```python
from build123d import *

# Parameters (mm, degrees)
F1_DEPTH = 28
F3_DEPTH = 72
F5_DEPTH = 28
F6_R     = 2
F7_R     = 1
F8_R     = 4.25
F9_DEPTH = 25


with BuildPart() as f1:
    # F0 (on Top) → F1 (new body)
    with BuildSketch(Plane.XY):
        Polygon((-19.75, -17.750001), (-19.75, -19.75), (-9.25, -19.75), (19.75, 9.25), (19.75, 19.75), (17.750001, 19.75), (17.750001, 10.078427), (-10.078427, -17.750001), align=None)
    extrude(amount=F1_DEPTH)

    # F2 (on face) → F3 (join)
    with BuildSketch(Plane.XY.offset(28)):
        Polygon((-19.75, -19.75), (-9.25, -19.75), (19.75, 9.25), (19.75, 19.75), (11.25, 19.75), (11.25, 24.25), (9.25, 26.25), (9.25, 23.421573), (9.25, 19.75), (9.25, 17.750001), (17.750001, 17.750001), (17.750001, 10.078427), (16.585787, 8.914213), (-8.914213, -16.585787), (-10.078427, -17.750001), (-17.750001, -17.750001), (-17.750001, -9.25), (-19.75, -9.25), (-23.421573, -9.25), (-26.25, -9.25), (-24.25, -11.25), (-19.75, -11.25), align=None)
    extrude(amount=F3_DEPTH)

    # F4 (on face) → F5 (join)
    with BuildSketch(Plane.XY.offset(100)):
        Polygon((19.75, 9.25), (19.75, 19.75), (17.750001, 19.75), (17.750001, 10.078427), (-10.078427, -17.750001), (-19.75, -17.750001), (-19.75, -19.75), (-9.25, -19.75), align=None)
    extrude(amount=F5_DEPTH)

    # F6
    f6_edges = [f1.edges().sort_by_distance(p)[0] for p in [
        (19.75, 9.25, 64),
        (-9.25, -19.75, 64),
    ]]
    fillet(f6_edges, radius=F6_R)

    # F7
    f7_edges = [f1.edges().sort_by_distance(p)[0] for p in [
        (-19.75, -19.75, 64),
        (19.75, 19.75, 64),
    ]]
    fillet(f7_edges, radius=F7_R)

    # F8 (on face) → F9 (cut)
    with BuildSketch(Plane(origin=(5.25, -5.25, 0), x_dir=(0.707107, 0.707107, 0), z_dir=(0.707107, -0.707107, 0))):
        with Locations((0, 114)):
            Circle(F8_R)
    extrude(amount=-F9_DEPTH, mode=Mode.SUBTRACT)


solid = f1.part
```
Check sheet for the modelled part. Datum: model origin and axes. Units: mm. A direction names the side the tool comes from. Round coordinates to 2 decimals unless told otherwise and drop trailing zeros. Write each loop counter-clockwise with the first axis right and the second up, starting at its lowest first coordinate (ties: lowest second). Pieces come first, ordered by that corner, then holes. Notation, with made-up numbers: (-33.5, 72.5) -> (-6.5, 72.5) arc R15 cw to (-6.5, 78.5) -> close; hole circle Ø3 at (39.5, 48). An arc over 180 degrees is marked (long way). Put each result on its own line as item: value.
(1) Sectioned sample at D-D (x = -16). Enter the section's corners in (y, z).
Values found:
outline: (-19.75, 0) -> (-17.75, 0) -> (-17.75, 128) -> (-19.75, 128) -> close
(2) Go/stop test with flat-tipped pins: pin 1 Ø9.5 at (y, z) = (-14, 53.5) entering from +X; pin 2 Ø5 at (x, z) = (-3, 88.5) entering from +Y; pin 3 Ø10.5 at (y, z) = (14.5, 69.5) entering from -X; pin 4 Ø8 at (x, y) = (11.5, 12) entering from -Z. Record where each tip stops, or that it passes through.
Values found:
pin 1: stops at x = 1.25
pin 2: stops at y = -8.17
pin 3: stops at x = 9.25
pin 4: passes through
(3) Tool access check on faces 5 (the face through (-19.75, -15, 63)), 6 (the face through (12.2, 19.5, 100)), 7 (the face through (11.25, 22, 63)). Record the directions out of +Z, -Z, +X, -X, +Y, -Y that give a thin tool (end or side, any length) a straight path to the whole face; none if there is none.
Values found:
face 5: +Z, -Z, -X, -Y
face 6: +Z, -X, +Y
face 7: +Z, -Z, +X, +Y
(4) Sectioned sample at C-C (z = 45.5). Enter the section's corners in (x, y).
Values found:
outline: (-26.25, -9.25) -> (-24.25, -11.25) -> (-19.75, -11.25) -> (-19.75, -18.75) arc R1 ccw to (-18.75, -19.75) -> (-10.08, -19.75) arc R2 ccw to (-8.66, -19.16) -> (19.16, 8.66) arc R2 ccw to (19.75, 10.08) -> (19.75, 18.75) arc R1 ccw to (18.75, 19.75) -> (11.25, 19.75) -> (11.25, 24.25) -> (9.25, 26.25) -> (9.25, 17.75) -> (17.75, 17.75) -> (17.75, 10.08) -> (-10.08, -17.75) -> (-17.75, -17.75) -> (-17.75, -9.25) -> close
(5) Material ranges on line 1 (X direction, y = 14, z = 36.5); line 2 (Y direction, x = -11, z = 118.5); line 3 (X direction, y = -15.5, z = 91), recorded low to high.
Values found:
line 1: x = 17.75 to 19.75
line 2: y = -19.75 to -17.75
line 3: x = -19.75 to -17.75, -7.83 to -5
(6) Mould release check, pull along Y, two halves, no side actions. Record for faces 1 (the face through (19.75, 14, 63)), 2 (the face through (-14, -19.75, 63)), 3 (the face through (13, 17.75, 63)), 4 (the face through (17.75, 15, 63)): released by +Y, released by -Y, zero draft, split by the parting line, or undercut.
Values found:
face 1: zero draft
face 2: released by -Y
face 3: undercut
face 4: undercut
(7) Sectioned sample at A-A (z = 13). Enter the section's corners in (x, y).
Values found:
outline: (-19.75, -18.75) arc R1 ccw to (-18.75, -19.75) -> (-10.08, -19.75) arc R2 ccw to (-8.66, -19.16) -> (19.16, 8.66) arc R2 ccw to (19.75, 10.08) -> (19.75, 18.75) arc R1 ccw to (18.75, 19.75) -> (17.75, 19.75) -> (17.75, 10.08) -> (-10.08, -17.75) -> (-19.75, -17.75) -> close
(8) Sectioned sample at B-B (x = 16). Enter the section's corners in (y, z).
Values found:
outline: (5.5, 0) -> (8.33, 0) -> (8.33, 128) -> (5.5, 128) -> close; (17.75, 28) -> (19.75, 28) -> (19.75, 100) -> (17.75, 100) -> close
